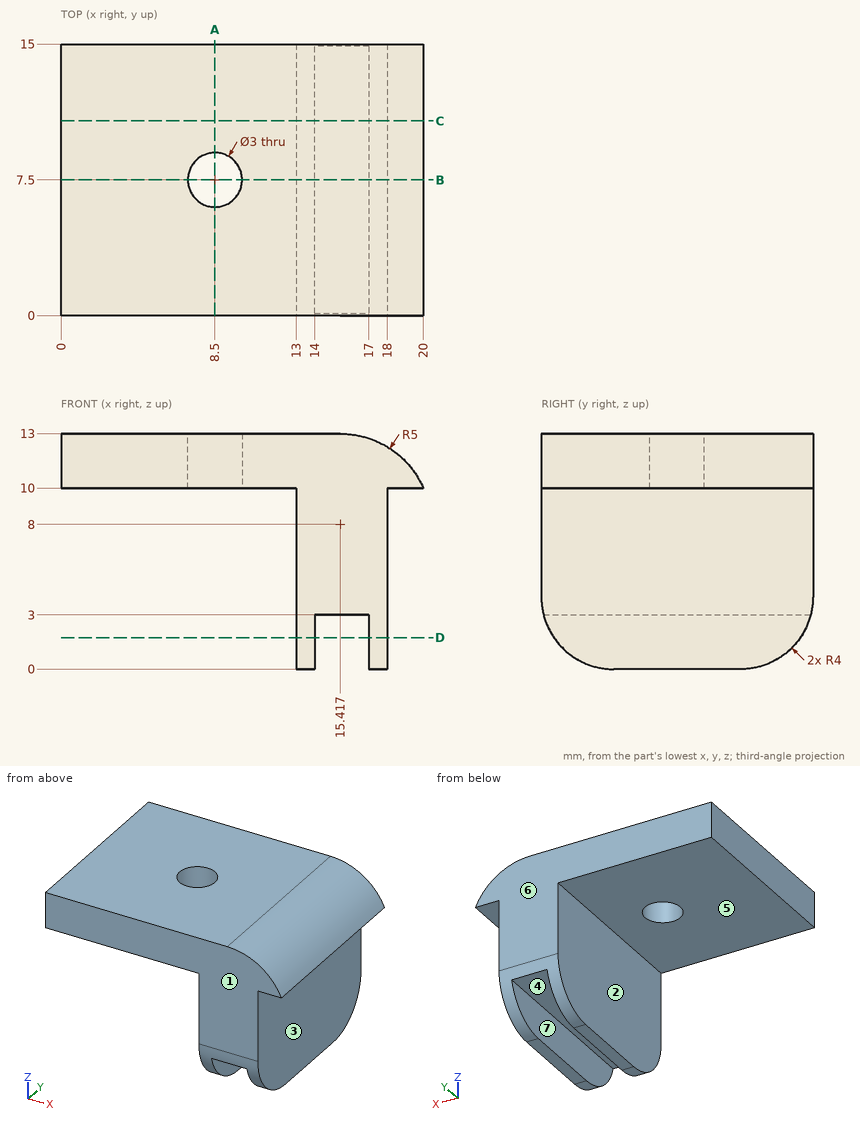
Part print with two shaded views. Sizes in mm from the minimum x, y, z corner. A direction names the side the tool comes from. Round coordinates to 2 decimals unless told otherwise and drop trailing zeros. Order: outer loops, then holes, each group sorted by start corner. A loop starts at its lowest first (then second) coordinate and runs counter-clockwise, first axis right, second up. Notation, with made-up numbers: (13.25, 24.5) -> (32.25, 24.5) arc R27 cw to (32.25, 46.5) -> close; hole circle Ø7 at (-18.5, -9). An arc over 180 degrees is marked (long way). Use one line per item in the form item = value.
Item 1: Pull direction X, two halves, no side cores. Call the marked faces 1, 2, 3 and 4: released by +X, released by -X, zero draft, split by the parting line, or undercut.
Returned:
face_1 = zero draft
face_2 = released by -X
face_3 = released by +X
face_4 = undercut
Item 2: Drill centre lines: line 1 (Y direction, x = 8.5, z = 10.8); line 2 (X direction, y = 3.25, z = 6.75); line 3 (Z direction, x = 12, y = 13.75). Where is each one in solid material? Low to high.
Returned:
line_1 = 0 to 6, 9 to 15
line_2 = 13 to 18
line_3 = 10 to 13
Item 3: Cut at C-C, the plane y = 10.75. Write the cut outline in (x, z).
Returned:
outline = (0, 10) -> (13, 10) -> (13, 0) -> (14, 0) -> (14, 3) -> (17, 3) -> (17, 0) -> (18, 0) -> (18, 10) -> (20, 10) arc R5 ccw to (15.42, 13) -> (0, 13) -> close
Item 4: Tool access for the marked faces 5, 6 and 7: list every direction of +Z, -Z, +X, -X, +Y, -Y with a clear straight run to the whole face (end or side of a thin tool).
Returned:
face_5 = -Z, -X, +Y, -Y
face_6 = +Z, -Z, +X, -X, +Y
face_7 = -Z, +Y, -Y
Item 5: Flat gauge pins, fed straight in: pin 1 Ø3 at (y, z) = (10.5, 5) entering from -X; pin 2 Ø0.6 at (x, y) = (19, 9.5) entering from -Z; pin 3 Ø1.5 at (x, y) = (15, 9.5) entering from -Z. Where does each tip first touch, or does it go through?
Returned:
pin_1 = 13
pin_2 = 10
pin_3 = 3
Item 6: Cut at D-D, the plane z = 1.75. Write the cut outline in (x, y).
Returned:
outline = (13, 0.69) -> (14, 0.69) -> (14, 14.31) -> (13, 14.31) -> close; (17, 0.69) -> (18, 0.69) -> (18, 14.31) -> (17, 14.31) -> close
Item 7: Cut at A-A, the plane x = 8.5. Write the cut outline in (y, z), and give its area (3 significant figures).
Returned:
outline = (0, 10) -> (6, 10) -> (6, 13) -> (0, 13) -> close; (9, 10) -> (15, 10) -> (15, 13) -> (9, 13) -> close
area = 36.0 mm^2
Item 8: Cut at B-B, the plane y = 7.5. Write the cut outline in (x, z).
Returned:
outline = (0, 10) -> (7, 10) -> (7, 13) -> (0, 13) -> close; (10, 10) -> (13, 10) -> (13, 0) -> (14, 0) -> (14, 3) -> (17, 3) -> (17, 0) -> (18, 0) -> (18, 10) -> (20, 10) arc R5 ccw to (15.42, 13) -> (10, 13) -> close
